Design review of the part built by this model. Coordinates are the model's own, in mm. Face numbers are marked on the shaded views. A direction names the side the tool comes from. Give positions to 0.01 mm unless a question says otherwise; leave off trailing zeros. Order: outer loops, then holes, each group sorted by start corner. A loop starts at its lowest first (then second) coordinate and runs counter-clockwise, first axis right, second up. Notation, with made-up numbers: (-35, 85) -> (1, 85) arc R30 ccw to (1, 110) -> close; hole circle Ø4 at (22, -25). An arc over 180 degrees is marked (long way). One line per item, written item: value. Start each with the question number.
1) For pin 1 (8 mm diameter, centred on x = -156.5, z = 305.5, fed in from +Y); pin 2 (8 mm diameter, centred on x = -192.5, z = 160, fed in from +Y), all flat-tipped, find the tip position at first contact; note any pin that passes through.
2) Wall thickness on line 1 along Z through (x, y) = (-324, 42); line 2 along Y through (x, z) = (-320, 580); line 3 along Z through (x, y) = (-60.5, -58.5): over which ranges is each line inside the solid? List them lowest first. Write a range as from..to.
3) Consider section A-A (y = -58.5). State the section outline as (x, z) points.
4) Consider section B-B (z = 661.5). State the section outline as (x, y) points.
5) The part is to be moulded in two halves that separate along Z. For the marked faces 3, 4, 5 and 6, say which applies: released by +Z, released by -Z, zero draft, split by the parting line, or undercut.
6) Tool access review of the marked faces 1 and 2: name each direction out of +Z, -Z, +X, -X, +Y, -Y from which nothing blocks a thin tool from reaching the whole face with its end or side.
7) Consider section C-C (x = -75.5). State the section outline as (y, z) points, plus the area to 3 significant figures.
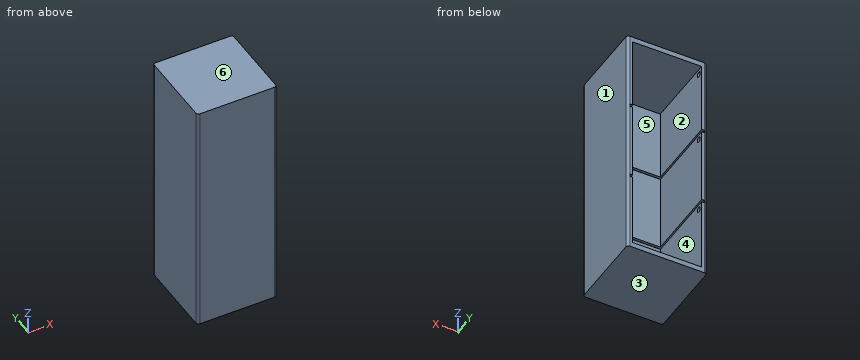
from build123d import *

# Parameters (mm, degrees)
SKETCH1_W           = 300
SKETCH1_H           = 300
BOSS_EXTRUDE1_DEPTH = 900
SHELL1_T            = -20
SKETCH2_W           = 280
SKETCH2_H           = 10
CUT_EXTRUDE1_DEPTH  = 290
SKETCH3_R           = 10
CUT_EXTRUDE2_DEPTH  = 10
FILLET1_START       = -1
FILLET1_DEPTH       = 902


with BuildPart() as part:
    # Sketch1 → Boss-Extrude1 (new body)
    with BuildSketch(Plane.XY):
        with Locations((-187.974683544, -55.696202532)):
            Rectangle(SKETCH1_W, SKETCH1_H)
    extrude(amount=BOSS_EXTRUDE1_DEPTH)

    # Shell1
    shell1_openings = [part.faces().sort_by_distance(p)[0] for p in [
        (-187.974683544, 94.303797468, 450),
    ]]
    offset(amount=SHELL1_T, openings=shell1_openings, kind=Kind.INTERSECTION)

    # Sketch2 → Cut-Extrude1 (cut)
    with BuildSketch(Plane(origin=(0, 94.303797468, 0), x_dir=(1, 0, 0), z_dir=(0, 1, 0))):
        with Locations((-187.974683544, -305)):
            Rectangle(SKETCH2_W, SKETCH2_H)
        with Locations((-187.974683544, -605)):
            Rectangle(SKETCH2_W, SKETCH2_H)
    extrude(amount=-CUT_EXTRUDE1_DEPTH, mode=Mode.SUBTRACT)

    # Sketch3 → Cut-Extrude2 (cut)
    with BuildSketch(Plane(origin=(-317.974683544, 0, 0), x_dir=(0, 0, -1), z_dir=(1, 0, 0))):
        with Locations(Location((-580, 74.303797468, 0), (0, 0, 90))):
            Circle(SKETCH3_R)
        with Locations(Location((-280, 74.303797468, 0), (0, 0, 90))):
            Circle(SKETCH3_R)
        with Locations(Location((-860, 74.303797468, 0), (0, 0, 90))):
            Circle(SKETCH3_R)
    extrude(amount=-CUT_EXTRUDE2_DEPTH, mode=Mode.SUBTRACT)

    # Fillet1: read off the stored shape, not the designer's step
    # Fillet1 outline → Fillet1 (cut)
    with BuildSketch(Plane.XY.offset(FILLET1_START)):
        with BuildLine():
            Line((-37.974683544, 94.303797468), (-47.974683544, 94.303797468))
            ThreePointArc((-47.974683544, 94.303797468), (-40.903615732, 91.37486528), (-37.974683544, 84.303797468))
            Line((-37.974683544, 84.303797468), (-37.974683544, 94.303797468))
        make_face()
        with BuildLine():
            Line((-37.974683544, -205.696202532), (-37.974683544, -195.696202532))
            ThreePointArc((-37.974683544, -195.696202532), (-40.903615732, -202.767270344), (-47.974683544, -205.696202532))
            Line((-47.974683544, -205.696202532), (-37.974683544, -205.696202532))
        make_face()
        with BuildLine():
            ThreePointArc((-337.974683544, 84.303797468), (-335.045751356, 91.37486528), (-327.974683544, 94.303797468))
            Line((-327.974683544, 94.303797468), (-337.974683544, 94.303797468))
            Line((-337.974683544, 94.303797468), (-337.974683544, 84.303797468))
        make_face()
        with BuildLine():
            Line((-337.974683544, -205.696202532), (-327.974683544, -205.696202532))
            ThreePointArc((-327.974683544, -205.696202532), (-335.045751356, -202.767270344), (-337.974683544, -195.696202532))
            Line((-337.974683544, -195.696202532), (-337.974683544, -205.696202532))
        make_face()
    extrude(amount=FILLET1_DEPTH, mode=Mode.SUBTRACT)


solid = part.part
Checked values:
1. pin 1: stops at y = -195.7
1. pin 2: stops at y = -185.7
2. line 1: z = 0..300, 310..600, 610..900
2. line 2: y = -205.7..64.3, 84.3..94.3
2. line 3: z = 0..20, 880..900
3. outline: (-337.97, 0) -> (-37.97, 0) -> (-37.97, 900) -> (-337.97, 900) -> close; hole (-327.97, 300) -> (-317.97, 300) -> (-317.97, 20) -> (-57.97, 20) -> (-57.97, 300) -> (-47.97, 300) -> (-47.97, 310) -> (-57.97, 310) -> (-57.97, 600) -> (-47.97, 600) -> (-47.97, 610) -> (-57.97, 610) -> (-57.97, 880) -> (-317.97, 880) -> (-317.97, 610) -> (-327.97, 610) -> (-327.97, 600) -> (-317.97, 600) -> (-317.97, 310) -> (-327.97, 310) -> close
4. outline: (-337.97, -195.7) arc R10 ccw to (-327.97, -205.7) -> (-47.97, -205.7) arc R10 ccw to (-37.97, -195.7) -> (-37.97, 84.3) arc R10 ccw to (-47.97, 94.3) -> (-57.97, 94.3) -> (-57.97, -185.7) -> (-317.97, -185.7) -> (-317.97, 94.3) -> (-327.97, 94.3) arc R10 ccw to (-337.97, 84.3) -> close
5. face 3: released by -Z
5. face 4: undercut
5. face 5: undercut
5. face 6: released by +Z
6. face 1: +Z, -Z, +X, +Y, -Y
6. face 2: +Y
7. outline: (-205.7, 0) -> (94.3, 0) -> (94.3, 20) -> (-185.7, 20) -> (-185.7, 300) -> (-195.7, 300) -> (-195.7, 310) -> (-185.7, 310) -> (-185.7, 600) -> (-195.7, 600) -> (-195.7, 610) -> (-185.7, 610) -> (-185.7, 880) -> (94.3, 880) -> (94.3, 900) -> (-205.7, 900) -> close
7. area: 29,000 mm^2
